Autodesk Inventor part; units mm, degrees
ref_plane "YZ Plane" through (0, 0, 0) normal (1, 0, 0) x (0, 1, 0)
ref_plane "XZ Plane" through (0, 0, 0) normal (0, 1, 0) x (-1, 0, 0)
ref_plane "XY Plane" through (0, 0, 0) normal (0, 0, 1) x (1, 0, 0)
sketch "スケッチ1" plane through (0, 0, 0) normal (0, 0, 1) x (1, 0, 0)
  line L0 (-47, 28.25) -> (-37.7144, 28.25)
  line L1 (47, 28.25) -> (47, 23.75)
  line L2 (47, -28.25) -> (-47, -28.25)
  line L3 (-47, -28.25) -> (-47, -11.5167)
  line L4 (-47, 28.25) -> (47, -28.25) construction
  line L5 (47, 28.25) -> (-47, -28.25) construction
  line L6 (0, 28.25) -> (0, -28.25) construction
  line L7 (-37.25, 9.4167) -> (-32.25, 9.4167) construction
  line L8 (-32.25, 9.4167) -> (-32.25, -9.4167) construction
  line L9 (-32.25, -9.4167) -> (-37.25, -9.4167) construction
  line L10 (-37.25, -9.4167) -> (-37.25, 9.4167) construction
  line L11 (-37.25, 9.4167) -> (-32.25, -9.4167) construction
  line L12 (-32.25, 9.4167) -> (-37.25, -9.4167) construction
  line L13 (-37.3, 9.4667) -> (-32.2, 9.4667)
  line L14 (-32.2, 9.4667) -> (-32.2, 7.3667) construction
  line L15 (-32.2, -9.4667) -> (-37.3, -9.4667)
  line L16 (-37.3, -9.4667) -> (-37.3, -7.3667) construction
  line L17 (-37.3, 9.4667) -> (-32.2, -9.4667) construction
  line L18 (-32.2, 9.4667) -> (-37.3, -9.4667) construction
  arc A0 (-37.3, 9.4667) -> (-37.3, 7.3667) centre (-37.3, 8.4167) ccw
  line L19 (-34.75, 9.4667) -> (-34.75, -9.4667) construction
  arc A1 (-32.2, 7.3667) -> (-32.2, 9.4667) centre (-32.2, 8.4167) ccw
  line L20 (-37.3, 7.3667) -> (-37.3, 9.4667) construction
  line L21 (-32.2, 7.3667) -> (-32.2, -7.3667)
  line L22 (-37.3, -7.3667) -> (-37.3, 7.3667)
  line L23 (-32.2, -7.3667) -> (-32.2, -9.4667) construction
  line L24 (37.25, 9.4167) -> (32.25, 9.4167) construction
  line L25 (32.25, 9.4167) -> (32.25, -9.4167) construction
  line L26 (32.25, -9.4167) -> (37.25, -9.4167) construction
  line L27 (37.25, -9.4167) -> (37.25, 9.4167) construction
  line L28 (37.25, 9.4167) -> (32.25, -9.4167) construction
  line L29 (32.25, 9.4167) -> (37.25, -9.4167) construction
  line L30 (37.3, 9.4667) -> (32.2, 9.4667)
  line L31 (32.2, 9.4667) -> (32.2, 7.3667) construction
  line L32 (32.2, -9.4667) -> (37.3, -9.4667)
  line L33 (37.3, -9.4667) -> (37.3, -7.3667) construction
  line L34 (37.3, 9.4667) -> (32.2, -9.4667) construction
  line L35 (32.2, 9.4667) -> (37.3, -9.4667) construction
  arc A2 (37.3, 7.3667) -> (37.3, 9.4667) centre (37.3, 8.4167) ccw
  line L36 (34.75, 9.4667) -> (34.75, -9.4667) construction
  arc A3 (32.2, 9.4667) -> (32.2, 7.3667) centre (32.2, 8.4167) ccw
  line L37 (37.3, 7.3667) -> (37.3, 9.4667) construction
  line L38 (32.2, 7.3667) -> (32.2, -7.3667)
  line L39 (37.3, -7.3667) -> (37.3, 7.3667)
  line L40 (32.2, -7.3667) -> (32.2, -9.4667) construction
  line L41 (-52, 9.4167) -> (-52, -9.4167)
  line L42 (-52, 9.4167) -> (-47, 9.4167)
  arc A4 (-47, 9.4167) -> (-47, 11.5167) centre (-47, 10.4667) ccw
  line L43 (-47, 11.5167) -> (-47, 23.75)
  line L44 (-47, -11.5167) -> (-47, 11.5167)
  line L45 (52, 9.4167) -> (52, -9.4167)
  line L46 (52, 9.4167) -> (47, 9.4167)
  arc A5 (47, 11.5167) -> (47, 9.4167) centre (47, 10.4667) ccw
  line L47 (47, 11.5167) -> (47, -11.5167)
  line L48 (47, -11.5167) -> (47, -28.25)
  line L49 (-52, 0) -> (52, 0) construction
  line L50 (-52, -9.4167) -> (-47, -9.4167)
  arc A6 (-47, -11.5167) -> (-47, -9.4167) centre (-47, -10.4667) ccw
  arc A7 (47, -9.4167) -> (47, -11.5167) centre (47, -10.4667) ccw
  line L51 (52, -9.4167) -> (47, -9.4167)
  line L52 (-37.3, 0) -> (-32.2, 0) construction
  arc A8 (-37.3, -7.3667) -> (-37.3, -9.4667) centre (-37.3, -8.4167) ccw
  arc A9 (-32.2, -9.4667) -> (-32.2, -7.3667) centre (-32.2, -8.4167) ccw
  arc A10 (32.2, -7.3667) -> (32.2, -9.4667) centre (32.2, -8.4167) ccw
  arc A11 (37.3, -9.4667) -> (37.3, -7.3667) centre (37.3, -8.4167) ccw
  arc A12 (-47, 24.0838) -> (-37.7144, 28.25) centre (-44.75, 31.5) ccw
  arc A13 (37.7144, 28.25) -> (47, 24.0838) centre (44.75, 31.5) ccw
  line L53 (-47, 24.0838) -> (-47, 28.25)
  line L54 (-37.7144, 28.25) -> (47, 28.25)
  arc A14 (-37.7144, 28.25) -> (-47, 24.0838) centre (-44.75, 31.5) ccw
  arc A15 (47, 24.0838) -> (37.7144, 28.25) centre (44.75, 31.5) ccw
  line L55 (-44.75, 23.75) -> (-47, 23.75)
  line L56 (44.75, 23.75) -> (47, 23.75)
  line L57 (-47, 23.75) -> (-47, 24.0838)
  line L58 (47, 23.75) -> (47, 11.5167)
  line L59 (-27.25, 23.25) -> (27.25, 23.25)
  line L60 (27.25, 23.25) -> (27.25, -23.25)
  line L61 (27.25, -23.25) -> (-27.25, -23.25)
  line L62 (-27.25, -23.25) -> (-27.25, 23.25)
  line L63 (-27.25, 23.25) -> (27.25, -23.25) construction
  line L64 (27.25, 23.25) -> (-27.25, -23.25) construction
  line L65 (-42, 8.25) -> (42, 8.25) construction
  line L66 (42, 8.25) -> (42, -18.25) construction
  line L67 (42, -18.25) -> (-42, -18.25) construction
  line L68 (-42, -18.25) -> (-42, 8.25) construction
  line L69 (-42, 8.25) -> (42, -18.25) construction
  line L70 (42, 8.25) -> (-42, -18.25) construction
  circle A16 centre (-39, 5.25) radius 1.25
  line L71 (-42, -5) -> (42, -5) construction
  circle A17 centre (-39, -15.25) radius 1.25
  circle A18 centre (39, 5.25) radius 1.25
  circle A19 centre (39, -15.25) radius 1.25
  point P0 (0, 0)
  point P1 (-34.75, 0)
  point P2 (34.75, 0)
  point P3 (0, 0)
  point P4 (-34.75, 0)
  point P5 (-34.75, 0)
  point P6 (0, 0)
  point P7 (0, 0)
  point P8 (47, 9.4167)
  point P9 (47, 9.4167)
  point P10 (0, -5)
  point P11 (0, -5)
  dimension "d57" = 90
  dimension "d0" = 94
  dimension "d1" = 56.5
  dimension "d2" = 5
  dimension "d3" = 18.8333
  dimension "d4" = 1.05
  dimension "d5" = 0.05
  dimension "d6" = 0.05
  dimension "d7" = 64.5
  dimension "d10" = 1.05
  dimension "d11" = 5
  dimension "d34" = 18.8333
  dimension "d40" = 31.5
  dimension "d41" = 89.5
  dimension "d42" = 15.5
  dimension "d43" = 52
  dimension "d60" = 5
  dimension "d63" = 5
  dimension "d69" = 5
  dimension "d70" = 20
  dimension "d71" = 10
  dimension "d72" = 84
  dimension "d73" = 26.5
  dimension "d78" = 2.5
  dimension "d80" = 3
  dimension "d81" = 3
extrude "押し出し1" add sketch "スケッチ1" along normal blind 5 contours L54 A13 L56 L58 A5 L47 A7 L48 L2 L3 A6 L44 A4 L43 L55 A12
extrude "押し出し2" add sketch "スケッチ1" along normal blind 2.5 contours L44 L50 L41 L42 | L46 L45 L51 L47
sketch "スケッチ2" plane through (47, 11.5167, 0) normal (1, 0, 0) x (0, 0, -1)
  line L0 (0, -23.0333) -> (-5, -23.0333)
  line L1 (-2.5, -23.0333) -> (-2.5, -39.7667)
  line L2 (0, -39.7667) -> (-5, -39.7667)
  line L3 (0, -2.1) -> (-2.5, -2.1)
  line L4 (0, -20.9333) -> (-2.5, -20.9333)
  point P0 (0, -11.5167)
  point P1 (-2.5, 7.9)
  dimension "d67" = 10
hole "穴1" at (47, 19.4167, 2.5) direction (-1, 0, 0) diameter 2.459 depth 10 tip angle 118
sketch "スケッチ3" plane through (-47, 11.5167, 0) normal (-1, 0, 0) x (0, 0, 1)
  circle A0 centre (2.5, 7.9) radius 1.2295
  circle A1 centre (2.5, -30.9333) radius 1.2295
  point P0 (0, -11.5167)
  point P1 (2.5, 7.9)
hole "穴2" at (-47, 19.4167, 2.5) direction (1, 0, 0) diameter 2.459 depth 10 tip angle 118
fillet "フィレット1" radius 1 4 edges at (-27.25, 23.25, 2.5) (-27.25, -23.25, 2.5) (27.25, -23.25, 2.5) (27.25, 23.25, 2.5)
equation "\"d3\" = d34"
equation "\"d6\" = d5"
equation "\"d10\" = d4"
properties part number "Cockpit_horizontal_frame_04" material "アセタール樹脂、黒"
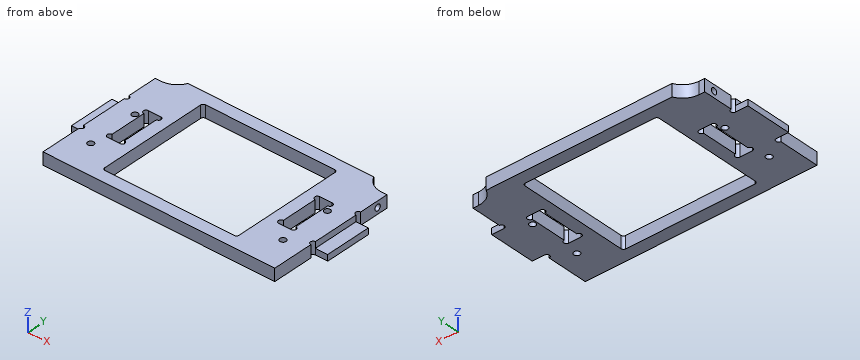
Build history of the part. All positions in model axes, mm. Round coordinates to 2 decimals unless told otherwise and drop trailing zeros. Write each loop counter-clockwise with the first axis right and the second up, starting at its lowest first coordinate (ties: lowest second). Pieces come first, ordered by that corner, then holes.
1) Drill centre lines: probe 1 along X at (y, z) = (-4, 3.7); probe 2 along X at (y, z) = (7, 1.3); probe 3 along Y at (x, z) = (6.5, 2.55). Where is each one in solid material? Low to high.
2) Band-saw the part on C-C, the plane y = 2. List the corners of the cut face in (x, z), and give its area (4 significant figures).
3) Band-saw the part on B-B, the plane x = 1.5. List the corners of the cut face in (y, z), and give its area (3 significant figures).
4) Pin check, flat tips, straight feed: pin 1 (2 mm diameter, centred on y = 19.42, z = 2.5, fed in from -X); pin 2 (4 mm diameter, centred on x = 50.5, y = 1, fed in from +Z); pin 3 (1.1 mm diameter, centred on x = 46, z = 3.5, fed in from +Y). Stop position of each tip, or through.
5) Band-saw the part on A-A, the plane y = -18. List the corners of the cut face in (x, z), and give its area (4 significant figures).
Ans:
1. probe 1: x = -47 to -37.3, -32.2 to -27.25, 27.25 to 32.2, 37.3 to 47
1. probe 2: x = -52 to -37.3, -32.2 to -27.25, 27.25 to 32.2, 37.3 to 52
1. probe 3: y = -28.25 to -23.25, 23.25 to 28.25
2. outline: (-52, 0) - (-37.3, 0) - (-37.3, 5) - (-47, 5) - (-47, 2.5) - (-52, 2.5) - close; (-32.2, 0) - (-27.25, 0) - (-27.25, 5) - (-32.2, 5) - close; (27.25, 0) - (32.2, 0) - (32.2, 5) - (27.25, 5) - close; (37.3, 0) - (52, 0) - (52, 2.5) - (47, 2.5) - (47, 5) - (37.3, 5) - close
2. area: 171.5 mm2
3. outline: (-28.25, 0) - (-23.25, 0) - (-23.25, 5) - (-28.25, 5) - close; (23.25, 0) - (28.25, 0) - (28.25, 5) - (23.25, 5) - close
3. area: 50.0 mm2
4. pin 1: stops at x = -36.86
4. pin 2: stops at z = 2.5
4. pin 3: stops at y = 23.75
5. outline: (-47, 0) - (-27.25, 0) - (-27.25, 5) - (-47, 5) - close; (27.25, 0) - (47, 0) - (47, 5) - (27.25, 5) - close
5. area: 197.5 mm2
